Autodesk Inventor part; units mm, degrees
ref_plane "Work Plane1" through (0, 16.5, 0) normal (0, 1, 0) x (1, 0, 0)
ref_plane "YZ Plane" through (0, 0, 0) normal (1, 0, 0) x (0, 1, 0)
ref_plane "XZ Plane" through (0, 0, 0) normal (0, 1, 0) x (-1, 0, 0)
sketch "Sketch1" plane through (0, 0, 0) normal (0, 1, 0) x (-1, 0, 0)
  line L0 (-21, 21) -> (21, 21)
  line L1 (21, 21) -> (21, -21)
  line L2 (21, -21) -> (-21, -21)
  line L3 (-21, -21) -> (-21, 21)
  line L4 (-21, 21) -> (21, -21) construction
  line L5 (21, 21) -> (-21, -21) construction
  point P0 (0, 0)
  dimension "d0" = 42
  dimension "d1" = 42
extrude "Extrusion1" add sketch "Sketch1" along normal blind 33
ref_plane "Work Plane1" through (0, 16.5, 0) normal (0, 1, 0) x (1, 0, 0)
sketch "Sketch2" plane through (0, 33, 0) normal (0, 1, 0) x (1, 0, 0)
  line L0 (0, -38.0423) -> (-38.0423, 0)
  line L1 (-38.0423, 0) -> (0, 38.0423)
  line L2 (0, 38.0423) -> (38.0423, 0)
  line L3 (38.0423, 0) -> (0, -38.0423)
  line L4 (0, -38.0423) -> (0, 38.0423) construction
  line L5 (-38.0423, 0) -> (38.0423, 0) construction
  line L6 (-21, 21) -> (-21, -21)
  circle A0 centre (0, 0) radius 250
  dimension "d4" = 53.8
  dimension "d5" = 53.8
  dimension "d6" = 500
extrude "Extrusion2" cut sketch "Sketch2" against normal blind 10
sketch "Sketch3" plane through (0, 16.5, 0) normal (0, 1, 0) x (1, 0, 0)
  line L0 (-20.9, -20.9) -> (20.9, -20.9)
  line L1 (20.9, -20.9) -> (20.9, 20.9)
  line L2 (20.9, 20.9) -> (-20.9, 20.9)
  line L3 (-20.9, 20.9) -> (-20.9, -20.9)
  line L4 (-21, -21) -> (-21, -17.0423)
  line L5 (21, -21) -> (17.0423, -21)
  line L6 (21, 21) -> (21, 17.0423)
  line L7 (-21, 21) -> (-17.0423, 21)
  circle A0 centre (0, 0) radius 200
  dimension "d9" = 0.1
  dimension "d10" = 0.1
  dimension "d11" = 0.1
  dimension "d12" = 0.1
  dimension "d13" = 400
extrude "Extrusion3" cut sketch "Sketch3" along normal up to surface (6.5 mm away)
chamfer "Chamfer1" distance 6 angle 45 4 edges at (20.9, 19.75, 20.9) (20.9, 19.75, -20.9) (-20.9, 19.75, 20.9) (-20.9, 19.75, -20.9)
mirror "Mirror1" about plane through (0, 16.5, 0) normal (0, 1, 0) of "Extrusion3", "Extrusion2", "Chamfer1"
sketch "Sketch4" plane through (0, 33, 0) normal (0, 1, 0) x (1, 0, 0)
  circle A0 centre (0, 0) radius 11
  dimension "d19" = 22
extrude "Extrusion4" add sketch "Sketch4" along normal blind 2
sketch "Sketch5" plane through (0, 33, 0) normal (0, 1, 0) x (1, 0, 0)
  circle A0 centre (0, 0) radius 11
  line L0 (17.0423, -21) -> (21, -17.0423)
  line L1 (21, -17.0423) -> (21, 17.0423)
  line L2 (21, 17.0423) -> (17.0423, 21)
  line L3 (17.0423, 21) -> (-17.0423, 21)
  line L4 (-17.0423, 21) -> (-21, 17.0423)
  line L5 (-21, 17.0423) -> (-21, -17.0423)
  line L6 (-21, -17.0423) -> (-17.0423, -21)
  line L7 (-17.0423, -21) -> (17.0423, -21)
  circle A1 centre (0, 0) radius 16
  dimension "d22" = 32
extrude "Extrusion5" cut sketch "Sketch5" against normal blind 0.5 contours A1
sketch "Sketch6" plane through (0, 35, 0) normal (0, 1, 0) x (1, 0, 0)
  circle A0 centre (0, 0) radius 3
  dimension "d25" = 6
extrude "Extrusion6" cut sketch "Sketch6" against normal blind 2
sketch "Sketch8" plane through (0, 33, 0) normal (0, 1, 0) x (1, 0, 0)
  circle A0 centre (0, 0) radius 16 construction
  line L0 (17.0423, -21) -> (21, -17.0423) construction
  line L1 (21, -17.0423) -> (21, 17.0423) construction
  line L2 (21, 17.0423) -> (17.0423, 21) construction
  line L3 (17.0423, 21) -> (-17.0423, 21) construction
  line L4 (-17.0423, 21) -> (-21, 17.0423) construction
  line L5 (-21, 17.0423) -> (-21, -17.0423) construction
  line L6 (-21, -17.0423) -> (-17.0423, -21) construction
  line L7 (-17.0423, -21) -> (17.0423, -21) construction
  line L8 (-15.5, -15.5) -> (15.5, -15.5) construction
  line L9 (15.5, -15.5) -> (15.5, 15.5) construction
  line L10 (15.5, 15.5) -> (-15.5, 15.5) construction
  line L11 (-15.5, 15.5) -> (-15.5, -15.5) construction
  line L12 (-15.5, -15.5) -> (15.5, 15.5) construction
  line L13 (15.5, -15.5) -> (-15.5, 15.5) construction
  circle A1 centre (-15.5, 15.5) radius 1.5
  circle A2 centre (15.5, 15.5) radius 1.5
  circle A3 centre (15.5, -15.5) radius 1.5
  circle A4 centre (-15.5, -15.5) radius 1.5
  dimension "d36" = 31
  dimension "d37" = 31
  dimension "d38" = 3
  dimension "d39" = 3
  dimension "d40" = 3
  dimension "d41" = 3
extrude "Extrusion8" cut sketch "Sketch8" against normal blind 5
thread "Thread2"
sketch "Sketch9" plane through (0, 33, 0) normal (0, 1, 0) x (1, 0, 0)
  circle A0 centre (0, 0) radius 2.5
  dimension "d49" = 5
extrude "Extrusion9" add sketch "Sketch9" along normal blind 20
pattern_circular "Circular Pattern2" count 4 over 360 about axis through (0, 33, 0) along (0, 1, 0) of "Extrusion8"
sketch "Sketch10" plane through (0, 53, 0) normal (0, 1, 0) x (1, 0, 0)
  circle A0 centre (0, 0) radius 2.5
  circle A1 centre (0, 0) radius 2.5
  line L0 (-1.5, -2) -> (1.5, -2)
  line L1 (1.5, -2) -> (1.5, -2.5)
  line L2 (1.5, -2.5) -> (-1.5, -2.5)
  line L3 (-1.5, -2.5) -> (-1.5, -2)
  circle A2 centre (0, 0) radius 2.5
  dimension "d55" = 0.5
extrude "Extrusion10" cut sketch "Sketch10" against normal blind 15 contours L0 A0 | A0 L2 L3 | L1 L2 A0 picked at (0.3466, -2.0912)
equation "\"d9\" = d10"
equation "\"d11\" = d10"
equation "\"d12\" = d10"
properties part number "nema17_33mm"
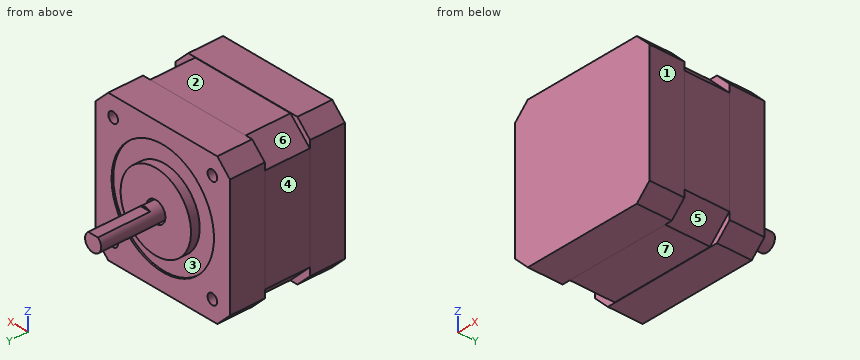
Verification items for the finished model (mm, model axes). Face numbers are marked on the shaded views. A direction names the side the tool comes from. Coordinates: 2 decimals unless noted, no trailing zeros. Loops run counter-clockwise (first coordinate to the right, second up) from the corner with the lowest first, then second, coordinate; pieces in that order, holes last. Notation, with made-up numbers: (54, 50.5) - (83, 50.5) arc R12 ccw to (83, 71.5) - close; hole circle Ø3 at (81, 49.5). An arc over 180 degrees is marked (long way). Answer as a JSON object with one key per item and string values.
(1) Access from +Z, -Z, +X, -X, +Y, -Y to the whole of each face (thin tool, end or side, straight path). Record for the marked faces 4, 5, 6 and 7.
Response:
{"face 4": "+Z, -Z, -X", "face 5": "-Z, +X", "face 6": "+Z, -X", "face 7": "-Z, +X, -X"}
(2) Go/stop test with flat-tipped pins: pin 1 Ø3.5 at (x, z) = (-16, -15.5) entering from +Y; pin 2 Ø0.9 at (x, y) = (0, 44.5) entering from +Z; pin 3 Ø4 at (x, y) = (9.5, 17) entering from -Z; pin 4 Ø8 at (y, z) = (42, -9) entering from +X. Record where each tip stops, or that it passes through.
Response:
{"pin 1": "stops at y = 33", "pin 2": "stops at z = 2", "pin 3": "stops at z = -20.9", "pin 4": "passes through"}
(3) Cross-section at A-A, the plane y = 3. Record the boundary of the cut face in (x, z).
Response:
{"outline": "(-21, -17.04) - (-17.04, -21) - (17.04, -21) - (21, -17.04) - (21, 17.04) - (17.04, 21) - (-17.04, 21) - (-21, 17.04) - close"}
(4) Scan lines: line 1 along Z through (x, y) = (0, 32.7); line 2 along Z through (x, y) = (-15.5, 31.5). Record each from-to range of solid material in increasing order.
Response:
{"line 1": "z = -21 to -16, -11 to 11, 16 to 21", "line 2": "z = -21 to -17, -14 to 14, 17 to 21"}
(5) Cross-section at C-C, the plane z = 0. Record the boundary of the cut face in (x, y).
Response:
{"outline": "(-21, 0) - (21, 0) - (21, 10) - (20.9, 10) - (20.9, 23) - (21, 23) - (21, 33) - (16, 33) - (16, 32.5) - (11, 32.5) - (11, 35) - (3, 35) - (3, 33) - (2.5, 33) - (2.5, 53) - (-2.5, 53) - (-2.5, 33) - (-3, 33) - (-3, 35) - (-11, 35) - (-11, 32.5) - (-16, 32.5) - (-16, 33) - (-21, 33) - (-21, 23) - (-20.9, 23) - (-20.9, 10) - (-21, 10) - close"}
(6) Cross-section at D-D, the plane y = 19. Record the boundary of the cut face in (x, z), then the cut area to 3 significant figures.
Response:
{"outline": "(-20.9, -14.9) - (-14.9, -20.9) - (14.9, -20.9) - (20.9, -14.9) - (20.9, 14.9) - (14.9, 20.9) - (-14.9, 20.9) - (-20.9, 14.9) - close", "area": "1,680 mm²"}
(7) Mould release check, pull along Y, two halves, no side actions. Record for the marked faces 1, 2 and 3: pulls with the +Y half, pulls with the -Y half, needs draft (parallel to the pull), parting line crosses it, or undercut.
Response:
{"face 1": "needs draft", "face 2": "undercut", "face 3": "pulls with the +Y half"}
